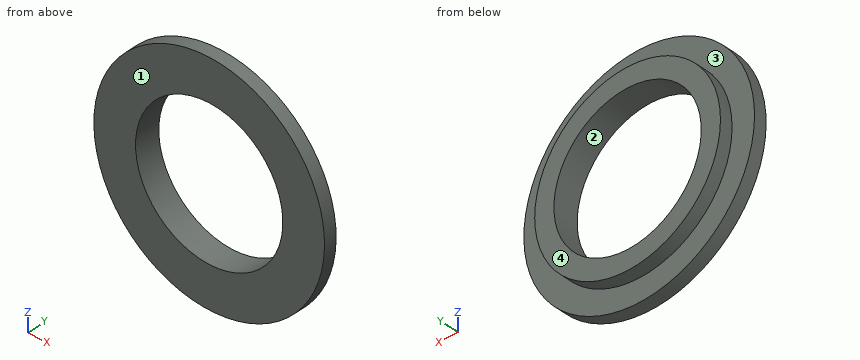
from build123d import *

# Parameters (mm, degrees)
SKETCH1_R               = 18
BOSS_EXTRUDE1_DEPTH     = 2
SKETCH2_R               = 14.5
BOSS_EXTRUDE2_DEPTH     = 2
CUT_EXTRUDE3_DEPTH      = 26.768197453
CUT_EXTRUDE3_DEPTH_BACK = 26.768197453
SKETCH3_R               = 11.5


with BuildPart() as part:
    # Sketch1 → Boss-Extrude1 (new body)
    with BuildSketch(Plane(origin=(0, 0, 0), x_dir=(1, 0, 0), z_dir=(0, 1, 0))):
        with Locations(Location((0, 0, 0), (0, 0, 270))):
            Circle(SKETCH1_R)
    extrude(amount=BOSS_EXTRUDE1_DEPTH)

    # Sketch2 → Boss-Extrude2 (add)
    with BuildSketch(Plane(origin=(0, 2, 0), x_dir=(1, 0, 0), z_dir=(0, 1, 0))):
        with Locations(Location((0, 0, 0), (0, 0, 270))):
            Circle(SKETCH2_R)
    extrude(amount=BOSS_EXTRUDE2_DEPTH)

    # Sketch3 → Cut-Extrude3 (cut, two sides: drawn at the far end of the back side and taken through both)
    with BuildSketch(Plane(origin=(0, 0, 0), x_dir=(1, 0, 0), z_dir=(0, 1, 0)).offset(-CUT_EXTRUDE3_DEPTH_BACK)):
        with Locations(Location((0, 0, 0), (0, 0, 270))):
            Circle(SKETCH3_R)
    extrude(amount=CUT_EXTRUDE3_DEPTH + CUT_EXTRUDE3_DEPTH_BACK, mode=Mode.SUBTRACT)


solid = part.part
Geometry: final body of the model. Coordinates: model frame, mm. Face numbers are marked on the shaded views. A direction names the side the tool comes from. Round coordinates to 2 decimals unless told otherwise and drop trailing zeros. Order: outer loops, then holes, each group sorted by start corner. A loop starts at its lowest first (then second) coordinate and runs counter-clockwise, first axis right, second up. Notation, with made-up numbers: (-37, 80) -> (-27, 80) arc R18 cw to (-27, 94) -> close; hole circle Ø3 at (9.25, 54). An arc over 180 degrees is marked (long way). Put each result on its own line as item: value. Start each with the question number.
Q1. Reachability of the marked faces 3 and 4 from +Z, -Z, +X, -X, +Y, -Y: full face, straight path, thin tool, end or side. Return the list, or none.
Q2. First-contact query: pin 1 (1 mm diameter, centred on y = 1, z = 3.5, fed in from +X); pin 2 (4 mm diameter, centred on x = -5.5, z = -14, fed in from +Y); pin 3 (1.5 mm diameter, centred on x = -14, y = 2.5, fed in from +Z); pin 4 (18.5 mm diameter, centred on x = 0, z = 0, fed in from -Y). Flat tips, straight axial feed; report the tip coordinate or a pass-through.
Q3. Section C-C on y = 3.45. Return the cut outline in (x, z).
Q4. Section A-A on x = 0. Return the cut outline in (y, z).
Q5. Section D-D on z = 13.5. Return the cut outline in (x, y), and give its area (3 significant figures).
Q6. Section B-B on z = 0. Return the cut outline in (x, y), and give its area (3 significant figures).
Q7. Line query: probe 1 along X at (y, z) = (2.7, 0); probe 2 along X at (y, z) = (1.15, 0); probe 3 along Y at (x, z) = (-2.5, 16). Output: solid intervals per line, ascending.
Q8. Pull-direction query (X, two-part tool) for the marked faces 1 and 2; classes: +X half, -X half, draft (parallel to the pull), parting line (faces both ways), or undercut.
Ans:
1. face 3: +Y
1. face 4: +Z, -Z, +X, -X, +Y
2. pin 1: stops at x = 17.75
2. pin 2: stops at y = 4
2. pin 3: stops at z = 11.97
2. pin 4: passes through
3. outline: circle Ø29 at (0, 0); hole circle Ø23 at (0, 0)
4. outline: (0, -18) -> (2, -18) -> (2, -14.5) -> (4, -14.5) -> (4, -11.5) -> (0, -11.5) -> close; (0, 11.5) -> (4, 11.5) -> (4, 14.5) -> (2, 14.5) -> (2, 18) -> (0, 18) -> close
5. outline: (-11.91, 0) -> (11.91, 0) -> (11.91, 2) -> (5.29, 2) -> (5.29, 4) -> (-5.29, 4) -> (-5.29, 2) -> (-11.91, 2) -> close
5. area: 68.8 mm2
6. outline: (-18, 0) -> (-11.5, 0) -> (-11.5, 4) -> (-14.5, 4) -> (-14.5, 2) -> (-18, 2) -> close; (11.5, 0) -> (18, 0) -> (18, 2) -> (14.5, 2) -> (14.5, 4) -> (11.5, 4) -> close
6. area: 38.0 mm2
7. probe 1: x = -14.5 to -11.5, 11.5 to 14.5
7. probe 2: x = -18 to -11.5, 11.5 to 18
7. probe 3: y = 0 to 2
8. face 1: draft
8. face 2: undercut
